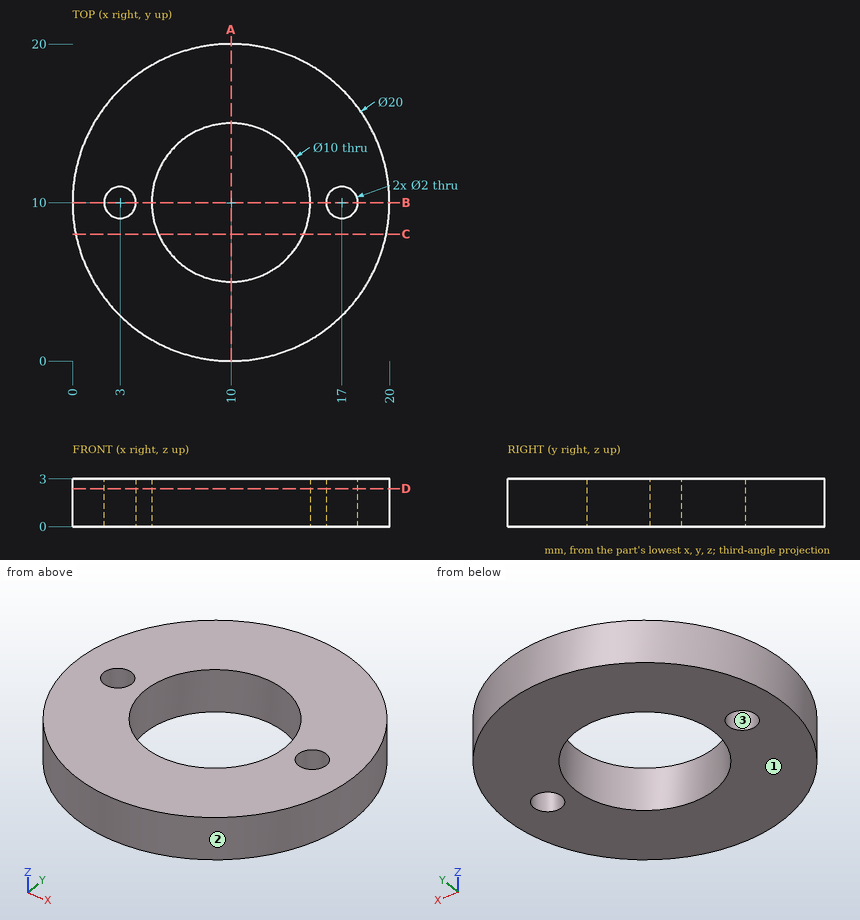
Input: dimensioned drawing with shaded views. Units: mm. Origin: part minimum x, y, z. Round coordinates to 2 decimals unless told otherwise and drop trailing zeros. Order: outer loops, then holes, each group sorted by start corner. A loop starts at its lowest first (then second) coordinate and runs counter-clockwise, first axis right, second up.
Q1. Section A-A, the plane x = 10. Output: boundary loops of the cut face in (y, z).
Result sheet:
outline: (0, 0) - (5, 0) - (5, 3) - (0, 3) - close; (15, 0) - (20, 0) - (20, 3) - (15, 3) - close
Q2. Material intervals for probe 1 along Y at (x, z) = (9.75, 0.25); probe 2 along X at (y, z) = (6.75, 1.1); probe 3 along Y at (x, z) = (3, 0.7), sorted ascending.
Result sheet:
probe 1: y = 0 to 5.01, 14.99 to 20
probe 2: x = 0.54 to 6.2, 13.8 to 19.46
probe 3: y = 2.86 to 9, 11 to 17.14
Q3. Mould query, pull axis Y, two halves, no side actions, for the marked faces 1, 2 and 3. Classes: released by +Y, released by -Y, zero draft, split by the parting line, or undercut.
Result sheet:
face 1: zero draft
face 2: split by the parting line
face 3: undercut
Q4. Section B-B, the plane y = 10. Output: boundary loops of the cut face in (x, z).
Result sheet:
outline: (0, 0) - (2, 0) - (2, 3) - (0, 3) - close; (4, 0) - (5, 0) - (5, 3) - (4, 3) - close; (15, 0) - (16, 0) - (16, 3) - (15, 3) - close; (18, 0) - (20, 0) - (20, 3) - (18, 3) - close
Q5. Pin query (flat end, axial travel): pin 1 (1 mm diameter, centred on y = 16, z = 2, fed in from +X); pin 2 (1 mm diameter, centred on x = 3.5, z = 2.5, fed in from -Y). Return the tip coordinate at first contact, or that it passes through.
Result sheet:
pin 1: stops at x = 18.35
pin 2: stops at y = 2
Q6. Section C-C, the plane y = 8. Output: boundary loops of the cut face in (x, z), and give its area (3 significant figures).
Result sheet:
outline: (0.2, 0) - (5.42, 0) - (5.42, 3) - (0.2, 3) - close; (14.58, 0) - (19.8, 0) - (19.8, 3) - (14.58, 3) - close
area: 31.3 mm2
Q7. Section D-D, the plane z = 2.4. Output: boundary loops of the cut face in (x, y).
Result sheet:
outline: circle Ø20 at (10, 10); hole circle Ø2 at (3, 10); hole circle Ø10 at (10, 10); hole circle Ø2 at (17, 10)
